CAD build for the part. Positions are in the model's coordinates, mm. A direction names the side the tool comes from. Give positions to 0.01 mm unless a question says otherwise; leave off trailing zeros. Loops run counter-clockwise (first coordinate to the right, second up) from the corner with the lowest first, then second, coordinate; pieces in that order, holes last.
Item 1: Drop flat-ended pins along their axis: P1, Ø10, axis at x = -13, y = 5.5, coming from the -Z side; P2, Ø2, axis at x = 10.5, z = -8, coming from the -Y side; P3, Ø2, axis at x = 14.5, z = -47, coming from the +Y side. Give the stop position or say it passes through.
Item 2: Probe probe 1 along Y at (x, z) = (30, 0); probe 2 along X at (y, z) = (47.5, 39); probe 3 along Y at (x, z) = (-0.5, 0) (3 decimals). List the from-to ranges inside material, lowest first.
Item 3: Mould opens along Y. For faces 1 (the cylindrical face through (-2.48, -24.98, 0.99)), 2 (the flat face through (-40, 21, 21)), 3 (the cylindrical face through (18.308, 105.432, -23.412)), 4 (the cylindrical face through (4.65, -30.04, 95.38)) say: released by +Y, released by -Y, zero draft, split by the parting line, or undercut.
Item 4: Saw through at B-B on y = 0. Give the number of separate pieces and of enclosed holes in the cut face, plus the area to 3 significant figures.
Item 5: Saw through at A-A on x = 10. Give the cut face in (y, z), plus the area to 3 significant figures.
Item 6: Saw through at D-D on x = -9. Give the cut face in (y, z), plus the area to 3 significant figures.
Item 7: Which spindle directions (+Z, -Z, +X, -X, +Y, -Y) get a long thin tool onto all of the face, cutting with end or side? Do faces 5 (the flat face through (34, -24, -8)), 6 (the cylindrical face through (27, 0, -82)), 7 (the flat face through (15, 43, 43)). Say none if no direction does.
from build123d import *

# Parameters (mm, degrees)
M16X2_0_TAPPED_HOLE1_D = 14
SKETCH4_W              = 21
SKETCH4_H              = 8
CUT_EXTRUDE1_DEPTH     = 8
CHAMFER2_SIZE          = 2
CUT_EXTRUDE2_START     = -11
SKETCH6_R              = 37.5
CUT_EXTRUDE2_DEPTH     = 11


with BuildPart() as part:
    # Sketch1 → Revolve1 (revolve)
    with BuildSketch(Plane.XY, mode=Mode.PRIVATE) as revolve1_sk:
        Polygon((-40, 25), (40, 25), (45, 25), (45, 37.5), (40, 37.5), (40, 108), (15, 108), (15, 50), (-40, 50), align=None)
    revolve(revolve1_sk.sketch.rotate(Axis((-40, 0, 0), (1, 0, 0)), 90), axis=Axis((-40, 0, 0), (1, 0, 0)))

    # M16x2.0 Tapped Hole1 (through all)
    with Locations(Plane(origin=(40, 0, 0), x_dir=(0, 0, -1), z_dir=(1, 0, 0))):
        with Locations((-75, 0), (0, 75), (75, 0), (0, -75)):
            Hole(M16X2_0_TAPPED_HOLE1_D / 2)

    # Sketch4 → Revolve2 (revolve)
    with BuildSketch(Plane.XY, mode=Mode.PRIVATE) as revolve2_sk:
        with Locations((4.5, 104)):
            Rectangle(SKETCH4_W, SKETCH4_H)
    revolve(revolve2_sk.sketch.rotate(Axis((0, 0, 0), (1, 0, 0)), 90), axis=Axis((0, 0, 0), (1, 0, 0)))

    # Sketch5 → Cut-Extrude1 (cut, symmetric)
    with BuildSketch(Plane.XY):
        Polygon((-40, 0), (45, 0), (45, 28.4), (-40, 27.55), align=None)
    extrude(amount=CUT_EXTRUDE1_DEPTH, both=True, mode=Mode.SUBTRACT)

    # Chamfer2
    chamfer2_edges = [part.edges().sort_by_distance(p)[0] for p in [
        (45, 0, -37.5),
        (-6, 0, -108),
        (-40, 0, -50),
        (15, 0, -50),
    ]]
    chamfer(chamfer2_edges, length=CHAMFER2_SIZE)

    # Sketch6 → Cut-Extrude2 (cut)
    with BuildSketch(Plane(origin=(45, 0, 0), x_dir=(0, 0, -1), z_dir=(1, 0, 0)).offset(CUT_EXTRUDE2_START)):
        Circle(SKETCH6_R)
    extrude(amount=CUT_EXTRUDE2_DEPTH, mode=Mode.SUBTRACT)


solid = part.part
Results below:
1. P1: stops at z = -50
1. P2: stops at y = -107.77
1. P3: stops at y = 97.71
2. probe 1: y = -108 to -82, -68 to -25, 28.25 to 68, 82 to 108
2. probe 2: x = 15 to 40
2. probe 3: y = -108 to -100, -50 to -25, 27.945 to 50, 100 to 108
3. face 1: undercut
3. face 2: zero draft
3. face 3: split by the parting line
3. face 4: undercut
4. separate pieces: 4
4. enclosed holes: 0
4. area: 6,380 mm2
5. outline: circle Ø216 at (0, 0); circle Ø100 at (0, 0); hole circle Ø200 at (0, 0); hole (23.69, -8) - (28.05, -8) - (28.05, 8) - (23.69, 8) arc R25 ccw (long way) to start
5. area: 11,100 mm2
6. outline: circle Ø100 at (0, 0); hole (23.69, -8) - (27.86, -8) - (27.86, 8) - (23.69, 8) arc R25 ccw (long way) to start
6. area: 5,840 mm2
7. face 5: +X
7. face 6: +X, -X
7. face 7: -X
